Check sheet for the modelled part. Datum: model origin and axes. Units: mm. Coordinates: 2 decimals unless noted, no trailing zeros. Write each loop counter-clockwise with the first axis right and the second up, starting at its lowest first coordinate (ties: lowest second). Pieces come first, ordered by that corner, then holes. Notation, with made-up numbers: (-20, 40) -> (22, 40) arc R12 cw to (22, 63) -> close; hole circle Ø7 at (0, 47). An arc over 180 degrees is marked (long way). One line per item, written item: value. Start each with the question number.
1) Draft check along Y on faces 1 (the flat face through (0, 4, 0)), 2 (the cylindrical face through (0, -2, 3)), 3 (the cylindrical face through (-14, 15, 3)), 4 (the cylindrical face through (-0.287, 11.207, 3.042)). Enter one of: +Y half, -Y half, draft (parallel to the pull), parting line (faces both ways), or undercut.
2) Scan lines: line 1 along Y through (x, z) = (0, 3.45) (3 decimals); line 2 along X through (y, z) = (-1.5, 4.5); line 3 along X through (y, z) = (-6.5, 1.5). Record each from-to range of solid material in increasing order. Write a range as [from, to].
3) Gauge pin test, flat end, axial feed: P1, Ø5, axis at x = -2, y = 2, coming from the -Z side. Record the tip position at first contact, or that the pin passes through.
4) Sectioned sample at B-B on z = 2.6. Enter the section's corners in (x, y) (3 decimals).
5) Sectioned sample at D-D on x = -11.5. Enter the section's corners in (y, z), plus the area to 3 significant figures.
6) Sectioned sample at C-C on y = -6.25. Enter the section's corners in (x, z).
7) Sectioned sample at A-A on y = 0. Enter the section's corners in (x, z).
Autodesk Inventor part; units mm, degrees
ref_plane "YZ Plane" through (0, 0, 0) normal (1, 0, 0) x (0, 1, 0)
ref_plane "XZ Plane" through (0, 0, 0) normal (0, 1, 0) x (-1, 0, 0)
ref_plane "XY Plane" through (0, 0, 0) normal (0, 0, 1) x (1, 0, 0)
sketch "Sketch1" plane through (0, 0, 0) normal (0, 0, 1) x (1, 0, 0)
  circle A0 centre (0, 0) radius 16 construction
  line L0 (-16, -16) -> (16, -16)
  line L1 (16, -16) -> (16, 16)
  line L2 (16, 16) -> (-16, 16)
  line L3 (-16, 16) -> (-16, -16)
  line L4 (-16, -16) -> (16, 16) construction
  line L5 (16, -16) -> (-16, 16) construction
  dimension "d0" = 32
extrude "Extrusion1" add sketch "Sketch1" along normal blind 6
sketch "Sketch2" plane through (0, 0, 6) normal (0, 0, 1) x (1, 0, 0)
  circle A0 centre (0, 0) radius 2
  dimension "d3" = 4
extrude "Extrusion2" cut sketch "Sketch2" against normal up to surface (6 mm away)
fillet "Fillet1" radius 5 4 edges at (16, 16, 3) (16, -16, 3) (-16, -16, 3) (-16, 16, 3)
sketch "Sketch3" plane through (0, 0, 6) normal (0, 0, 1) x (1, 0, 0)
  circle A0 centre (0, 0) radius 2 construction
  circle A1 centre (0, 0) radius 12.5 construction
  line L0 (0, -22.4) -> (0, 22.4) construction
  line L1 (-22.4, 0) -> (22.4, 0) construction
  circle A2 centre (0, 12.5) radius 1.325
  circle A3 centre (10.8253, -6.25) radius 1.325
  circle A4 centre (-10.8253, -6.25) radius 1.325
  line L2 (0, 0) -> (22.5547, -13.0219) construction
  line L3 (0, 0) -> (-20.3118, -11.727) construction
  dimension "d7" = 25
  dimension "d8" = 2.65
  dimension "d9" = 2.65
  dimension "d10" = 2.65
  dimension "d11" = 30
  dimension "d12" = 30
extrude "Extrusion3" cut sketch "Sketch3" against normal through all
equation "\"d9\" = d8"
equation "\"d10\" = d8"
properties part number "MiddleStandOff"
Answers:
1. face 1: draft
1. face 2: undercut
1. face 3: +Y half
1. face 4: undercut
2. line 1: y = [-16, -2], [2, 11.175], [13.825, 16]
2. line 2: x = [-16, -1.32], [1.32, 16]
2. line 3: x = [-16, -12.13], [-9.52, 9.52], [12.13, 16]
3. P1: stops at z = 0
4. outline: (-16, -11) arc R5 ccw to (-11, -16) -> (11, -16) arc R5 ccw to (16, -11) -> (16, 11) arc R5 ccw to (11, 16) -> (-11, 16) arc R5 ccw to (-16, 11) -> close; hole circle Ø2.65 at (-10.825, -6.25); hole circle Ø4 at (0, 0); hole circle Ø2.65 at (0, 12.5); hole circle Ø2.65 at (10.825, -6.25)
5. outline: (-15.97, 0) -> (-7.39, 0) -> (-7.39, 6) -> (-15.97, 6) -> close; (-5.11, 0) -> (15.97, 0) -> (15.97, 6) -> (-5.11, 6) -> close
5. area: 178 mm2
6. outline: (-16, 0) -> (-12.15, 0) -> (-12.15, 6) -> (-16, 6) -> close; (-9.5, 0) -> (9.5, 0) -> (9.5, 6) -> (-9.5, 6) -> close; (12.15, 0) -> (16, 0) -> (16, 6) -> (12.15, 6) -> close
7. outline: (-16, 0) -> (-2, 0) -> (-2, 6) -> (-16, 6) -> close; (2, 0) -> (16, 0) -> (16, 6) -> (2, 6) -> close
